CAD build for the part. Positions are in the model's coordinates, mm. Face numbers are marked on the shaded views. Give positions to 0.01 mm unless a question says otherwise; leave off trailing zeros. Order: outer loops, then holes, each group sorted by start corner. A loop starts at its lowest first (then second) coordinate and runs counter-clockwise, first axis right, second up.
Item 1: Two-plate mould, pull along Y, no slides. Class the marked faces 1 and 2: released by +Y, released by -Y, zero draft, split by the parting line, or undercut.
Item 2: Wall check: L1, parallel to Y at x = 0, z = 27.1; L2, parallel to Y at x = -0.95, z = 27; L3, parallel to X at y = 1.4, z = 20.25. Give the ranges that are in metal, low to high.
Item 3: Flat gauge pin, fed straight in: P1, Ø1.5, axis at x = 0, y = 0, coming from the -Z side. Where does the tip first touch, or does it go through?
Item 4: Band-saw the part on B-B on z = 22. Give the cut face in (x, y), plus the area to 3 significant figures.
Item 5: Band-saw the part on C-C on y = 1.55. Give the cut face in (x, z).
Item 6: Band-saw the part on A-A on z = 4.5. Give the cut face in (x, y).
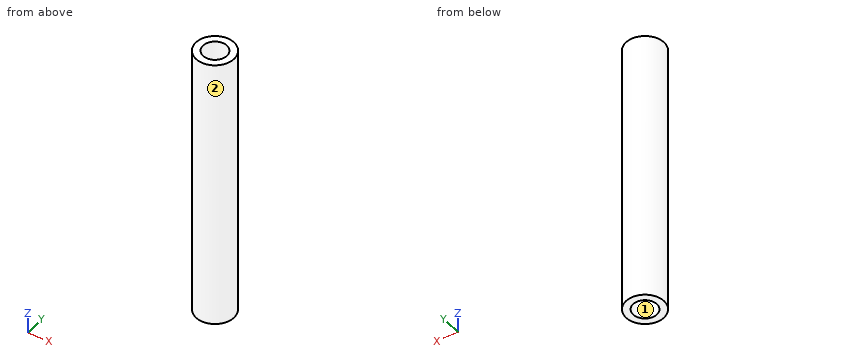
```python
from build123d import *

# Parameters (mm, degrees)
SKETCH1_R           = 2
BOSS_EXTRUDE1_DEPTH = 29


with BuildPart() as part:
    # Sketch1 → Boss-Extrude1 (new body)
    with BuildSketch(Plane.XY):
        with Locations(Location((0, 0, 0), (0, 0, 180))):
            Circle(SKETCH1_R)
    extrude(amount=BOSS_EXTRUDE1_DEPTH)

    # Sketch6 → Tap Drill for M3x0.5 Tap1 (revolve, cut)
    with BuildSketch(Plane(origin=(0, 0, 29), x_dir=(0, -1, 0), z_dir=(1, 0, 0))):
        Polygon((0, 0), (0, 5.751075774), (1.25, 5), (1.25, 0), align=None)
    tap_drill_for_m3x0_5_tap1 = revolve(axis=Axis((0, 0, 35.35), (0, 0, -1)), mode=Mode.SUBTRACT)

    # Mirror2: Tap Drill for M3x0.5 Tap1 across plane
    add(tap_drill_for_m3x0_5_tap1.mirror(Plane(origin=(0, 0, 14.5), x_dir=(1, 0, 0), z_dir=(0, 0, -1))), mode=Mode.SUBTRACT)


solid = part.part
```
The answers:
1. face 1: undercut
1. face 2: split by the parting line
2. L1: y = -2 to -1.25, 1.25 to 2
2. L2: y = -1.76 to -0.81, 0.81 to 1.76
2. L3: x = -1.43 to 1.43
3. P1: stops at z = 5.3
4. outline: circle Ø4 at (0, 0)
4. area: 12.6 mm2
5. outline: (-1.26, 0) - (1.26, 0) - (1.26, 29) - (-1.26, 29) - close
6. outline: circle Ø4 at (0, 0); hole circle Ø2.5 at (0, 0)
